CAD build for the part. Positions are in the model's coordinates, mm. A direction names the side the tool comes from. Give positions to 0.01 mm unless a question says otherwise; leave off trailing zeros. Write each loop counter-clockwise with the first axis right and the second up, starting at its lowest first coordinate (ties: lowest second). Pieces come first, ordered by that corner, then holes. Notation, with made-up numbers: (-29, 78) - (-11, 78) arc R37 cw to (-11, 117) - close; hole circle Ø3 at (85, 19.25). An arc over 180 degrees is marked (long way). Put each result on its own line as item: value. Start each with the question number.
1. Cut at A-A on z = 5. List the corners of the cut face in (x, y).
2. Mould opens along Y. For faces 4 (the cylindrical face through (-22.498, 0.07, 5.185)), 5 (the cylindrical face through (-1.5, 0.07, 4.96)), 6 (the cylindrical face through (3, 4, 5)) say: +Y half, -Y half, draft (parallel to the pull), parting line (faces both ways), or undercut.
3. Cut at B-B on x = -15. List the corners of the cut face in (y, z).
4. Cut at C-C on y = 0. List the corners of the cut face in (x, z).
5. Drop flat-ended pins along their axis: pin 1 (6 mm diameter, centred on y = 3.5, z = 4.5, fed in from -X); pin 2 (2 mm diameter, centred on y = 1, z = 3, fed in from -X); pin 3 (3 mm diameter, centred on x = -8.5, y = 0.5, fed in from -Z); pin 4 (4 mm diameter, centred on x = -15, z = 5, fed in from +Y). Give the stop position or say it passes through.
6. Wall check: line 1 (Y direction, x = 0, z = 3.75); line 2 (Z direction, x = -15, y = 3.25); line 3 (X direction, y = 0, z = 6.4). Give the ranges that are in metal, low to high.
7. Tool access for faces 1 (the flat face through (-3, 0, 7.5)), 2 (the cylindrical face through (3, -4, 5)), 3 (the flat face through (-3, 0, 2.5)): list every direction of +Z, -Z, +X, -X, +Y, -Y with a clear straight run to the whole face (end or side of a thin tool).
8. Cut at D-D on y = 4. List the corners of the cut face in (x, z).
from build123d import *

# Parameters (mm, degrees)
CROQUIS1_W              = 25
CROQUIS1_H              = 10
CROQUIS1_R              = 1.5
SALIENTE_EXTRUIR1_DEPTH = 10
CROQUIS2_R              = 2.5
CORTAR_EXTRUIR1_DEPTH   = 14
CROQUIS3_OUTSIDE_W      = 17.744
CROQUIS3_OUTSIDE_H      = 17.744
CROQUIS3_OUTSIDE_W_2    = 5
CROQUIS3_OUTSIDE_H_2    = 10
CORTAR_EXTRUIR2_DEPTH   = 12.5
CUT_EXTRUDE1_DEPTH      = 10
CROQUIS5_R              = 2.5
SALIENTE_EXTRUIR5_DEPTH = 10
CORTAR_EXTRUIR3_DEPTH   = 28.613402543


with BuildPart() as part:
    # Croquis1 → Saliente-Extruir1 (new body)
    with BuildSketch(Plane.XY):
        with Locations((-7.5, 0)):
            Rectangle(CROQUIS1_W, CROQUIS1_H)
        Circle(CROQUIS1_R, mode=Mode.SUBTRACT)
    extrude(amount=SALIENTE_EXTRUIR1_DEPTH)

    # Croquis2 → Cortar-Extruir1 (cut)
    with BuildSketch(Plane(origin=(0, 5, 0), x_dir=(1, 0, 0), z_dir=(0, 1, 0))):
        with Locations(Location((-15, -5, 0), (0, 0, 180))):
            Circle(CROQUIS2_R)
    extrude(amount=-CORTAR_EXTRUIR1_DEPTH, mode=Mode.SUBTRACT)

    # Croquis3 outside → Cortar-Extruir2 (cut)
    with BuildSketch(Plane(origin=(5, 0, 0), x_dir=(0, 0, -1), z_dir=(1, 0, 0))):
        with Locations((-5, 0)):
            Rectangle(CROQUIS3_OUTSIDE_W, CROQUIS3_OUTSIDE_H)
        with Locations((-5, 0)):
            Rectangle(CROQUIS3_OUTSIDE_W_2, CROQUIS3_OUTSIDE_H_2, mode=Mode.SUBTRACT)
    extrude(amount=-CORTAR_EXTRUIR2_DEPTH, mode=Mode.SUBTRACT)

    # Sketch1 → Cut-Extrude1 (cut)
    with BuildSketch(Plane.XY.offset(10)):
        with BuildLine():
            Line((0, 5), (5.992915048, 5))
            Line((5.992915048, 5), (5.992915048, -6.748814934))
            Line((5.992915048, -6.748814934), (0, -5))
            ThreePointArc((0, -5), (2.680080756, -4.221038633), (4.525089765, -2.126866856))
            Line((4.525089765, -2.126866856), (4.525089765, 2.126866856))
            ThreePointArc((4.525089765, 2.126866856), (2.680080756, 4.221038633), (0, 5))
        make_face()
    extrude(amount=-CUT_EXTRUDE1_DEPTH, mode=Mode.SUBTRACT)

    # Croquis5 → Saliente-Extruir5 (add)
    with BuildSketch(Plane(origin=(0, 5, 0), x_dir=(1, 0, 0), z_dir=(0, 1, 0))):
        with BuildLine():
            Line((-12.115384615, 1.923076923), (-7.5, 0))
            Line((-7.5, 0), (-7.5, -10))
            Line((-7.5, -10), (-11.574224798, -11.67188611))
            ThreePointArc((-11.574224798, -11.67188611), (-22.494065139, -5.298308051), (-12.115384615, 1.923076923))
        make_face()
        with Locations(Location((-15, -5, 0), (0, 0, 180))):
            Circle(CROQUIS5_R, mode=Mode.SUBTRACT)
    extrude(amount=-SALIENTE_EXTRUIR5_DEPTH)

    # Croquis6 → Cortar-Extruir3 (cut, through all)
    with BuildSketch(Plane(origin=(0, 5, 0), x_dir=(1, 0, 0), z_dir=(0, 1, 0))):
        Polygon((-13.556059362, 2.359689901), (-7.5, -2.5), (-7.5, 2.359689901), align=None)
        Polygon((-7.5, -7.5), (-7.5, -12.359689901), (-13.556059362, -12.359689901), align=None)
    extrude(amount=-CORTAR_EXTRUIR3_DEPTH, mode=Mode.SUBTRACT)


solid = part.part
Report:
1. outline: (-22.5, -5) - (-17.5, -5) - (-17.5, 5) - (-22.5, 5) - close; (-12.5, -5) - (0, -5) arc R5 ccw to (4.53, -2.13) - (4.53, 2.13) arc R5 ccw to (0, 5) - (-12.5, 5) - close; hole circle Ø3 at (0, 0)
2. face 4: draft
2. face 5: undercut
2. face 6: +Y half
3. outline: (-5, -2.5) - (5, -2.5) - (5, 2.5) - (-5, 2.5) - close; (-5, 7.5) - (5, 7.5) - (5, 12.5) - (-5, 12.5) - close
4. outline: (-13.56, -2.36) - (-7.5, 2.5) - (-1.5, 2.5) - (-1.5, 7.5) - (-7.5, 7.5) - (-13.56, 12.36) arc R7.5 ccw (long way) to start; (1.5, 2.5) - (4.53, 2.5) - (4.53, 7.5) - (1.5, 7.5) - close; hole circle Ø5 at (-15, 5)
5. pin 1: stops at x = -22.5
5. pin 2: stops at x = -22.43
5. pin 3: stops at z = 0.49
5. pin 4: passes through
6. line 1: y = -5 to -1.5, 1.5 to 5
6. line 2: z = -2.5 to 2.5, 7.5 to 12.5
6. line 3: x = -22.37 to -17.07, -12.93 to -1.5, 1.5 to 4.53
7. face 1: +Z, +X, +Y, -Y
7. face 2: +Z, -Z, +X, -Y
7. face 3: -Z, +X, +Y, -Y
8. outline: (-13.56, -2.36) - (-7.5, 2.5) - (3, 2.5) - (3, 7.5) - (-7.5, 7.5) - (-13.56, 12.36) arc R7.5 ccw (long way) to start; hole circle Ø5 at (-15, 5)
